Design review of the part built by this model. Coordinates are the model's own, in mm. Face numbers are marked on the shaded views. Round coordinates to 2 decimals unless told otherwise and drop trailing zeros. Order: outer loops, then holes, each group sorted by start corner. A loop starts at its lowest first (then second) coordinate and runs counter-clockwise, first axis right, second up.
from build123d import *

# Parameters (mm, degrees)
F0_W     = 200
F0_H     = 100
F1_DEPTH = 30
F3_SIZE2 = 10
F3_SIZE  = 10
F2_R     = 7.5
F2_R_2   = 15
F2_R_3   = 22.5
F4_DEPTH = 30.001


with BuildPart() as f1:
    # F0 (on Top) → F1 (new body)
    with BuildSketch(Plane.XY):
        Rectangle(F0_W, F0_H)
    extrude(amount=F1_DEPTH)

    # F3
    f3_edges = [f1.edges().sort_by_distance(p)[0] for p in [
        (0, -50, 30),
        (100, 0, 30),
        (0, 50, 30),
        (-100, 0, 30),
        (0, -50, 0),
        (100, 0, 0),
        (-100, 0, 0),
        (0, 50, 0),
    ]]
    chamfer(f3_edges, length=F3_SIZE, length2=F3_SIZE2)

    # F2 (on face) → F4 (cut, through all)
    with BuildSketch(Plane.XY.offset(30)):
        with Locations((-75, 0)):
            Circle(F2_R)
        with Locations((-25, 0)):
            Circle(F2_R_2)
        with Locations((50, 0)):
            Circle(F2_R_3)
    extrude(amount=-F4_DEPTH, mode=Mode.SUBTRACT)


solid = f1.part
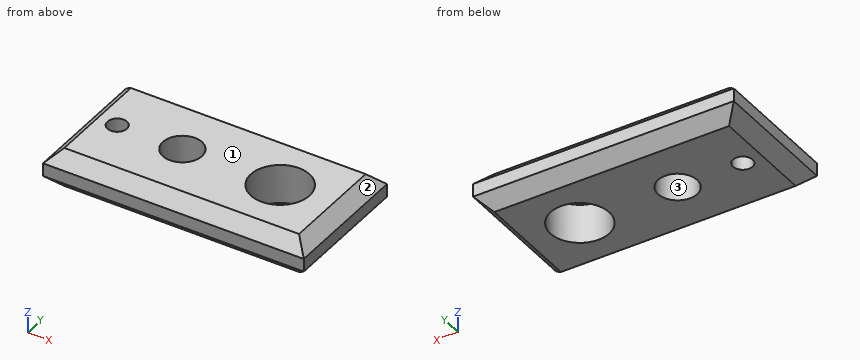
1) Take a section at D-D on y = -30. Give the boundary of the cut face in (x, z).
Results:
outline: (-100, 10) - (-90, 0) - (90, 0) - (100, 10) - (100, 20) - (90, 30) - (-90, 30) - (-100, 20) - close
2) The part is to be moulded in two halves that separate along X. For the marked faces 1, 2 and 3, say which applies: released by +X, released by -X, zero draft, split by the parting line, or undercut.
Results:
face 1: zero draft
face 2: released by +X
face 3: undercut
3) Take a section at A-A on y = 0. Give the boundary of the cut face in (x, z).
Results:
outline: (-100, 10) - (-90, 0) - (-82.5, 0) - (-82.5, 30) - (-90, 30) - (-100, 20) - close; (-67.5, 0) - (-40, 0) - (-40, 30) - (-67.5, 30) - close; (-10, 0) - (27.5, 0) - (27.5, 30) - (-10, 30) - close; (72.5, 0) - (90, 0) - (100, 10) - (100, 20) - (90, 30) - (72.5, 30) - close
4) Take a section at C-C on z = 6.5. Give the boundary of the cut face in (x, y), plus the area to 3 significant figures.
Results:
outline: (-96.5, -46.5) - (96.5, -46.5) - (96.5, 46.5) - (-96.5, 46.5) - close; hole circle Ø15 at (-75, 0); hole circle Ø30 at (-25, 0); hole circle Ø45 at (50, 0)
area: 15,500 mm2
5) Clearance check with a flat-ended pin moving along its axis: P1, Ø1.5, axis at x = 67, z = 26, coming from the -Y side. State where the tip first meets the part, or that it passes through.
Results:
P1: stops at y = -44.75
6) To check wall thickness, follow line 1 along X through (y, z) = (-0.5, 12.5); line 2 along Y through (x, z) = (-75, 18); line 3 along Y through (x, z) = (-25, 11). State the ranges of each line that lie inside material, in increasing order.
Results:
line 1: x = -100 to -82.48, -67.52 to -39.99, -10.01 to 27.51, 72.49 to 100
line 2: y = -50 to -7.5, 7.5 to 50
line 3: y = -50 to -15, 15 to 50
7) Take a section at B-B on x = -25. Give the boundary of the cut face in (y, z).
Results:
outline: (-50, 10) - (-40, 0) - (-15, 0) - (-15, 30) - (-40, 30) - (-50, 20) - close; (15, 0) - (40, 0) - (50, 10) - (50, 20) - (40, 30) - (15, 30) - close
